Part model, mm, in its own coordinate system. Round coordinates to 2 decimals unless told otherwise and drop trailing zeros. Write each loop counter-clockwise with the first axis right and the second up, starting at its lowest first coordinate (ties: lowest second). Pieces come first, ordered by that corner, then holes. Notation, with made-up numbers: M 10,63.5 L 31,63.5 A31 cw 31,92.5 Z; hole C 52,3 d3. An arc over 180 degrees is marked long. Use a Markdown table: item, result. Add a question column.
1) Slice it at C-C on z = 2.5. Write the cut outline in (x, y).
2) Slice it at D-D on z = -25. Write the cut outline in (x, y), plus the area to 3 significant figures.
3) Wall check: probe 1 along Z at (x, y) = (53, 12.5); probe 2 along Y at (x, z) = (-0.5, -26); probe 3 along X at (y, z) = (9.5, 18.5). Give the ranges that are in metal, low to high.
4) Drop flat-ended pins along their axis: P1, Ø0.9, axis at y = 10, z = 31.5, coming from the +X side; P2, Ø2, axis at x = 60, y = 49.5, coming from the -Z side; P3, Ø4.5, axis at x = 52.5, z = -12.5, coming from the +Y side; P4, Ø2, axis at x = 59.5, y = 49.5, coming from the +Z side. Give the stop position or say it passes through.
5) Slice it at A-A on z = -7.5. Write the cut outline in (x, y), plus the area to 3 significant figures.
6) Slice it at B-B on x = 38. Write the cut outline in (y, z), plus the area to 3 significant figures.
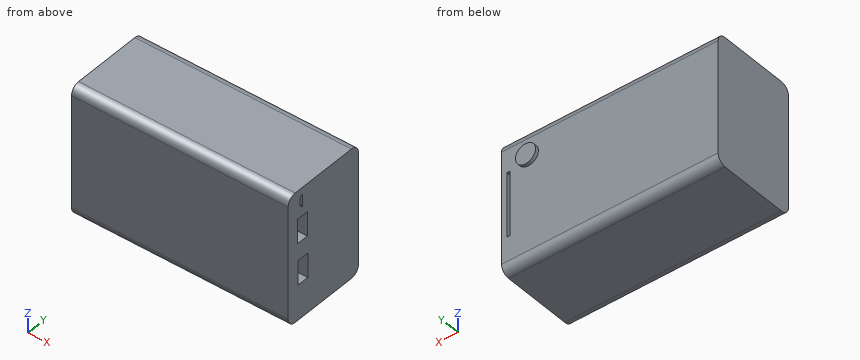
```python
from build123d import *

# Parameters (mm, degrees)
F0_W      = 127
F0_H      = 76.2
F1_DEPTH  = 50.8
F2_R      = 5.08
F3_W      = 7
F3_H      = 14.3
F4_DEPTH  = 16.4
F5_W      = 7
F5_H      = 14.3
F6_DEPTH  = 16.4
F8_DEPTH  = 16.4
F9_W      = 1.841523
F9_H      = 37.853485
F10_DEPTH = 3
F11_R     = 5.920901
F12_DEPTH = 2


with BuildPart() as f1:
    # F0 (on Front) → F1 (new body)
    with BuildSketch(Plane.XZ):
        Rectangle(F0_W, F0_H)
    extrude(amount=-F1_DEPTH)

    # F2
    f2_edges = [f1.edges().sort_by_distance(p)[0] for p in [
        (0, 50.8, -38.1),
        (0, 0, -38.1),
        (0, 0, 38.1),
        (0, 50.8, 38.1),
    ]]
    fillet(f2_edges, radius=F2_R)

    # F3 (on face) → F4 (cut)
    with BuildSketch(Plane.YZ.offset(63.5)):
        with Locations((10.331045, 14.323671)):
            Rectangle(F3_W, F3_H)
    extrude(amount=-F4_DEPTH, mode=Mode.SUBTRACT)

    # F5 (on face) → F6 (cut)
    with BuildSketch(Plane.YZ.offset(63.5)):
        with Locations((10.71509, -10.272532)):
            Rectangle(F5_W, F5_H)
    extrude(amount=-F6_DEPTH, mode=Mode.SUBTRACT)

    # F7 (on face) → F8 (cut)
    with BuildSketch(Plane.YZ.offset(63.5)):
        with BuildLine():
            Line((10.417472, 33.898923), (10.367472, 33.898923))
            ThreePointArc((10.367472, 33.898923), (9.09468, 33.371715), (8.567472, 32.098923))
            Line((8.567472, 32.098923), (8.567472, 28.798923))
            ThreePointArc((8.567472, 28.798923), (9.09468, 27.526131), (10.367472, 26.998923))
            Line((10.367472, 26.998923), (10.417472, 26.998923))
            Line((10.417472, 26.998923), (10.417472, 33.898923))
        make_face()
    extrude(amount=-F8_DEPTH, mode=Mode.SUBTRACT)

    # F9 (on face) → F10 (cut)
    with BuildSketch(Plane(origin=(0, 50.8, 0), x_dir=(-1, 0, 0), z_dir=(0, 1, 0))):
        with Locations((-59.478882, 0.321649)):
            Rectangle(F9_W, F9_H)
    extrude(amount=-F10_DEPTH, mode=Mode.SUBTRACT)

    # F11 (on face) → F12 (join)
    with BuildSketch(Plane(origin=(0, 50.8, 0), x_dir=(-1, 0, 0), z_dir=(0, 1, 0))):
        with Locations((-47.834026, 22.763033)):
            Circle(F11_R)
    extrude(amount=F12_DEPTH)


solid = f1.part
```
Entries:
| question | item | result |
|---|---|---|
| 1 | outline | M -63.5,0 L 63.5,0 L 63.5,50.8 L 60.4,50.8 L 60.4,47.8 L 58.56,47.8 L 58.56,50.8 L -63.5,50.8 Z |
| 2 | outline | M -63.5,0 L 63.5,0 L 63.5,50.8 L -63.5,50.8 Z |
| 2 | area | 6,450 mm^2 |
| 3 | probe 1 | z = -38.1 to -17.42, -3.12 to 7.17, 21.47 to 38.1 |
| 3 | probe 2 | y = 0 to 50.8 |
| 3 | probe 3 | x = -63.5 to 47.1 |
| 4 | P1 | stops at x = 63.5 |
| 4 | P2 | stops at z = -37.27 |
| 4 | P3 | stops at y = 50.8 |
| 4 | P4 | stops at z = 37.27 |
| 5 | outline | M -63.5,0 L 63.5,0 L 63.5,7.22 L 47.1,7.22 L 47.1,14.22 L 63.5,14.22 L 63.5,50.8 L 60.4,50.8 L 60.4,47.8 L 58.56,47.8 L 58.56,50.8 L -63.5,50.8 Z |
| 5 | area | 6,330 mm^2 |
| 6 | outline | M 0,-33.02 A5.08 ccw 5.08,-38.1 L 45.72,-38.1 A5.08 ccw 50.8,-33.02 L 50.8,33.02 A5.08 ccw 45.72,38.1 L 5.08,38.1 A5.08 ccw 0,33.02 Z |
| 6 | area | 3,850 mm^2 |
